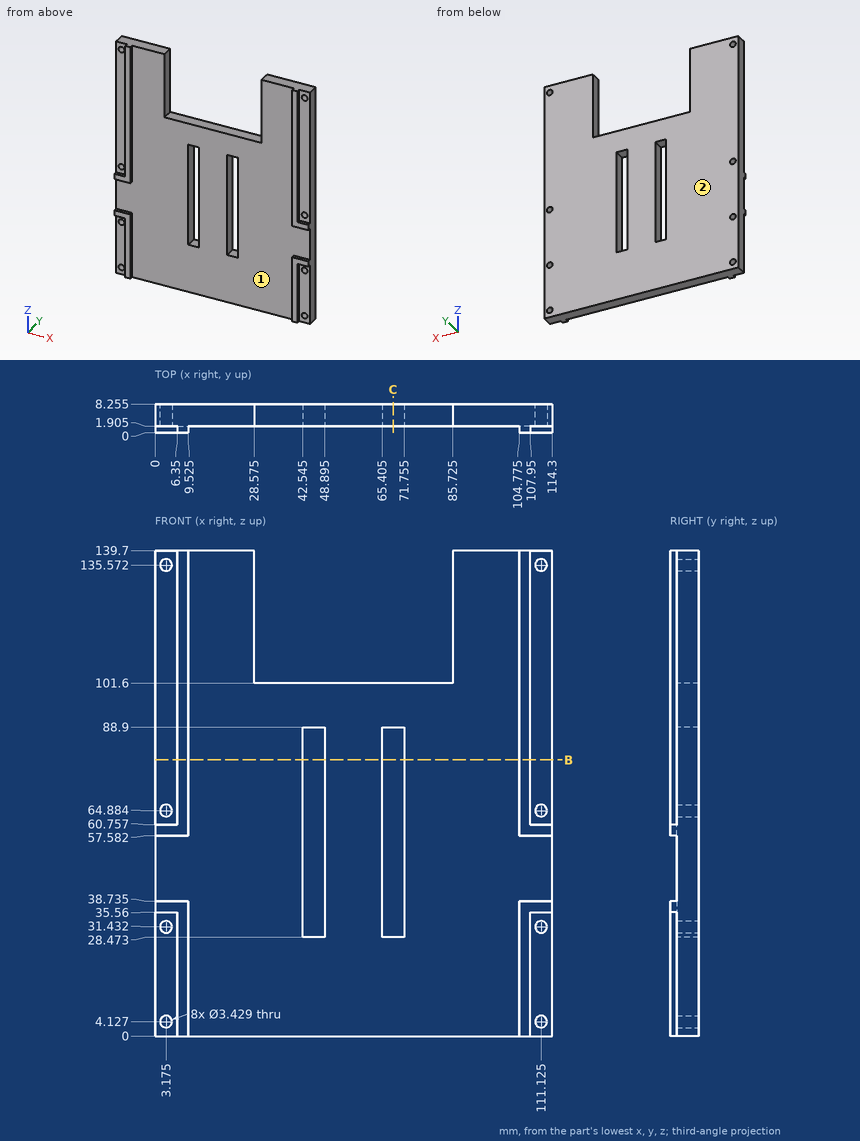
Source: three-view drawing plus pictorial views. Frame: mm from the lowest corner of the part. Coordinates: 2 decimals unless noted, no trailing zeros. Order: outer loops, then holes, each group sorted by start corner. A loop starts at its lowest first (then second) coordinate and runs counter-clockwise, first axis right, second up. Notation, with made-up numbers: M -23.5,12.25 L 32.5,12.25 A23 ccw 32.5,42.25 Z; hole C 86,-14 d3. An arc over 180 degrees is marked long. One line per question, with ' | ' between items. Start each with the question number.
Item 1: Pin query (flat end, axial travel): pin 1 Ø12 at (x, z) = (73.5, 63) entering from -Y (1 decimal); pin 2 Ø0.6 at (x, y) = (111, 1.5) entering from -Z; pin 3 Ø4 at (x, y) = (47, 6) entering from +Z. Return the tip coordinate at first contact, or that it passes through.
Item 2: Cut plane B-B, the plane z = 79.5. Count the separate pieces of the cut face and the enclosed holes in it.
Item 3: Cut plane C-C, the plane x = 68.5. Return the cut outline in (y, z) (1 decimal).
Item 4: Draft query along X for the marked faces 1 and 2. Return one class per face: released by +X, released by -X, zero draft, split by the parting line, or undercut.
Item 5: Ray query, probe 1 along X at (y, z) = (7.5, 87) (1 decimal); probe 2 along X at (y, z) = (6, 114) (1 decimal); probe 3 along Z at (x, y) = (81, 2.75). Return the intervals inside material, ascending. Write a range as [from, to].
A:
1) pin 1: stops at y = 1.9 | pin 2: stops at z = 35.56 | pin 3: stops at z = 101.6
2) separate pieces: 3 | enclosed holes: 0
3) outline: M 1.9,0 L 8.3,0 L 8.3,28.5 L 1.9,28.5 Z; M 1.9,88.9 L 8.3,88.9 L 8.3,101.6 L 1.9,101.6 Z
4) face 1: undercut | face 2: zero draft
5) probe 1: x = [0, 42.5], [48.9, 65.4], [71.8, 114.3] | probe 2: x = [0, 28.6], [85.7, 114.3] | probe 3: z = [0, 101.6]
